Part model, mm, in its own coordinate system. A direction names the side the tool comes from. Give positions to 0.01 mm unless a question says otherwise; leave off trailing zeros. Order: outer loops, then holes, each group sorted by start corner. A loop starts at its lowest first (then second) coordinate and runs counter-clockwise, first axis right, second up.
1. Slice it at B-B on y = -375. List the corners of the cut face in (x, z).
2. Drop flat-ended pins along their axis: pin 1 Ø1 at (x, z) = (1, -7) entering from -Y; pin 2 Ø1.5 at (x, z) = (-2, -8) entering from +Y; pin 3 Ø6.5 at (y, z) = (-364.82, -7.5) entering from -X. Give the stop position or say it passes through.
3. Mould opens along Y. For faces 1 (the flat face through (-13.192, -381.475, -7.395)), 2 (the cylindrical face through (1.56, -377.74, -7.4)), 3 (the flat face through (1, -375.373, -8)) say: +Y half, -Y half, draft (parallel to the pull), parting line (faces both ways), or undercut.
4. Slice it at D-D on z = -12.25. List the corners of the cut face in (x, y).
5. Probe line 1 (Y direction, x = 0.95, z = -7.5); line 2 (Y direction, x = 1.15, z = -7.5); line 3 (X direction, y = -360, z = -13). List the from-to ranges inside material, lowest first.
6. Slice it at C-C on y = -365.5. List the corners of the cut face in (x, z), and give its area (3 significant figures).
7. Slice it at A-A on z = -7.5. List the corners of the cut face in (x, y).
8. Which spindle directions (+Z, -Z, +X, -X, +Y, -Y) get a long thin tool onto all of the face, cutting with end or side? Do faces 4 (the flat face through (1, -373.273, -8)), 5 (the flat face through (0, -368, -7)), 6 (the cylindrical face through (1.01, -356.82, -1.43)). Say none if no direction does.
from build123d import *

# Parameters (mm, degrees)
DODANIE_WYCI_GNI_CIE1_DEPTH = 15
SZKIC2_R                    = 2.5
WYTNIJ_WYCI_GNI_CIE3_DEPTH  = 15
SZKIC4_W                    = 5.1
SZKIC4_H                    = 2.1
WYTNIJ_WYCI_GNI_CIE8_DEPTH  = 15
ZAOKR_GLENIE1_R             = 5


with BuildPart() as part:
    # Szkic1 → Dodanie-wyciągnięcie1 (new body)
    with BuildSketch(Plane.XY):
        with BuildLine():
            Line((0.355050358, -378.672211739), (-25.016650403, -387.906755609))
            Line((-25.016650403, -387.906755609), (-25.70069069, -386.027370367))
            Line((-25.70069069, -386.027370367), (-0.328989928, -376.792826498))
            ThreePointArc((-0.328989928, -376.792826498), (-0.090423978, -376.609768405), (0, -376.322980187))
            Line((0, -376.322980187), (0, -375.320100819))
            Line((0, -375.320100819), (0, -373.324775164))
            Line((0, -373.324775164), (0, -360.320100819))
            Line((0, -360.320100819), (0, -355.320100819))
            Line((0, -355.320100819), (2, -355.320100819))
            Line((2, -355.320100819), (2, -360.320100819))
            Line((2, -360.320100819), (2, -375.320100819))
            Line((2, -375.320100819), (2, -376.322980187))
            ThreePointArc((2, -376.322980187), (1.547880111, -377.756921278), (0.355050358, -378.672211739))
        make_face()
    extrude(amount=-DODANIE_WYCI_GNI_CIE1_DEPTH)

    # Szkic2 → Wytnij-wyciągnięcie3 (cut)
    with BuildSketch(Plane(origin=(2, 0, 0), x_dir=(0, 0, -1), z_dir=(1, 0, 0))):
        with Locations((7.5, -364.820100819)):
            Circle(SZKIC2_R)
    extrude(amount=-WYTNIJ_WYCI_GNI_CIE3_DEPTH, mode=Mode.SUBTRACT)

    # Szkic4 → Wytnij-wyciągnięcie8 (cut)
    with BuildSketch(Plane(origin=(2, 0, 0), x_dir=(0, 0, -1), z_dir=(1, 0, 0))):
        with Locations((7.55, -374.322980187)):
            Rectangle(SZKIC4_W, SZKIC4_H)
    extrude(amount=-WYTNIJ_WYCI_GNI_CIE8_DEPTH, mode=Mode.SUBTRACT)

    # Zaokrąglenie1
    zaokr_glenie1_edges = [part.edges().sort_by_distance(p)[0] for p in [
        (1, -355.320100819, -15),
        (1, -355.320100819, 0),
    ]]
    fillet(zaokr_glenie1_edges, radius=ZAOKR_GLENIE1_R)


solid = part.part
Data:
1. outline: (0, -15) - (2, -15) - (2, -10.1) - (0, -10.1) - close; (0, -5) - (2, -5) - (2, 0) - (0, 0) - close
2. pin 1: stops at y = -378.61
2. pin 2: stops at y = -377.13
2. pin 3: stops at x = 0
3. face 1: +Y half
3. face 2: -Y half
3. face 3: undercut
4. outline: (-25.7, -386.03) - (-25.02, -387.91) - (0.36, -378.67) arc R2.5 ccw to (2, -376.32) - (2, -355.85) - (0, -355.85) - (0, -376.32) arc R0.5 cw to (-0.33, -376.79) - close
5. line 1: y = -378.36 to -375.37, -373.27 to -367.32, -362.32 to -355.32
5. line 2: y = -378.2 to -375.37, -373.27 to -367.32, -362.32 to -355.32
5. line 3: x = 0 to 2
6. outline: (0, -15) - (2, -15) - (2, -9.91) - (0, -9.91) - close; (0, -5.09) - (2, -5.09) - (2, 0) - (0, 0) - close
6. area: 20.4 mm2
7. outline: (-25.7, -386.03) - (-25.02, -387.91) - (0.36, -378.67) arc R2.5 ccw to (2, -376.32) - (2, -375.37) - (0, -375.37) - (0, -376.32) arc R0.5 cw to (-0.33, -376.79) - close; (0, -373.27) - (2, -373.27) - (2, -367.32) - (0, -367.32) - close; (0, -362.32) - (2, -362.32) - (2, -355.32) - (0, -355.32) - close
8. face 4: +X, -X
8. face 5: +Z, -Z, -X, +Y
8. face 6: +Z, +X, -X, +Y
